Part print with two shaded views. Sizes in mm from the minimum x, y, z corner. A direction names the side the tool comes from. Give positions to 0.01 mm unless a question says otherwise; leave off trailing zeros. Order: outer loops, then holes, each group sorted by start corner. A loop starts at its lowest first (then second) coordinate and runs counter-clockwise, first axis right, second up. Notation, with made-up numbers: (-39, 44.5) - (-8, 44.5) arc R16 cw to (-8, 62.5) - close; hole circle Ø4 at (45, 89). An arc over 180 degrees is marked (long way). Return JSON: item names as keys, results as strings. Group by question number.
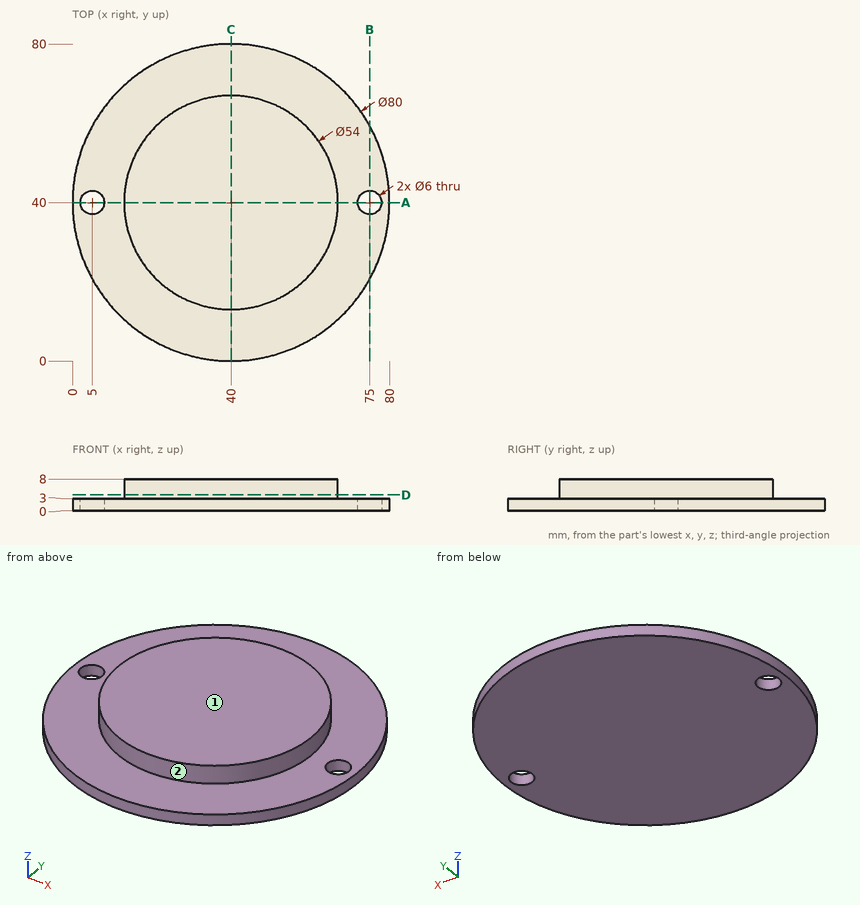
(1) Slice it at B-B (x = 75). Give the cut face in (y, z), and give its area (3 significant figures).
(2) Slice it at A-A (y = 40). Give the cut face in (x, z).
(3) Drill centre lines: L1, parallel to Z at x = 11, y = 13.5; L2, parallel to Y at x = 75, z = 1.45; L3, parallel to X at y = 51.5, z = 5.75. Where is each one in solid material? Low to high.
(4) 3-axis set-ups, long thin cutter, end or side, ignore diameter. For the marked faces 1 and 2: which of +Z, -Z, +X, -X, +Y, -Y reach the whole face in a straight line?
(5) Slice it at C-C (x = 40). Give the cut face in (y, z).
(6) Drop flat-ended pins along their axis: pin 1 Ø8 at (x, y) = (5, 40) entering from -Z; pin 2 Ø1.5 at (y, z) = (43, 7) entering from -X; pin 3 Ø1 at (y, z) = (53.5, 2.5) entering from +X; pin 4 Ø2 at (x, z) = (59.5, 4.5) entering from +Y. Give the stop position or say it passes through.
(7) Slice it at D-D (z = 4). Give the cut face in (x, y).
Result set:
{
 "1": {"outline": "(20.64, 0) - (37, 0) - (37, 3) - (20.64, 3) - close; (43, 0) - (59.36, 0) - (59.36, 3) - (43, 3) - close", "area": "98.2 mm²"},
 "2": {"outline": "(0, 0) - (2, 0) - (2, 3) - (0, 3) - close; (8, 0) - (72, 0) - (72, 3) - (67, 3) - (67, 8) - (13, 8) - (13, 3) - (8, 3) - close; (78, 0) - (80, 0) - (80, 3) - (78, 3) - close"},
 "3": {"L1": "z = 0 to 3", "L2": "y = 20.64 to 37, 43 to 59.36", "L3": "x = 15.57 to 64.43"},
 "4": {"face 1": "+Z, +X, -X, +Y, -Y", "face 2": "+Z"},
 "5": {"outline": "(0, 0) - (80, 0) - (80, 3) - (67, 3) - (67, 8) - (13, 8) - (13, 3) - (0, 3) - close"},
 "6": {"pin 1": "stops at z = 0", "pin 2": "stops at x = 13.09", "pin 3": "stops at x = 77.83", "pin 4": "stops at y = 59.67"},
 "7": {"outline": "circle Ø54 at (40, 40)"}
}
